Check sheet for the drawn part. Datum: minimum x, y, z corner. Units: mm. A direction names the side the tool comes from. Coordinates: 2 decimals unless noted, no trailing zeros. Order: outer loops, then holes, each group sorted by start corner. A loop starts at its lowest first (then second) coordinate and runs counter-clockwise, first axis right, second up. Notation, with made-up numbers: (0, 19.25) - (4, 19.25) arc R22 cw to (4, 39.25) - close; hole circle Ø7 at (0.5, -8). An arc over 180 degrees is marked (long way). Answer as CSV lines item,"result". Start each with the question number.
1. Section check A-A (x = 6). Record the cut outline in (y, z).
2. Section check C-C (x = 15). Record the cut outline in (y, z).
3. Section check D-D (z = 36). Record the cut outline in (x, y), and give its area (3 significant figures).
4. Section check B-B (y = 17.5). Record the cut outline in (x, z).
5. Set-up check for the marked faces 1 and 2: record each of +Z, -Z, +X, -X, +Y, -Y from which the full face is reachable in a straight line by a thin tool's end or side.
6. Material ranges on L1, parallel to Y at x = 6, z = 46.15; L2, parallel to Z at x = 4, y = 21; L3, parallel to X at y = 29, z = 46, recorded low to high. Write a range as [from, to].
7. Go/stop test with flat-tipped pins: pin 1 (6 mm diameter, centred on x = 19.5, z = 33, fed in from +Y); pin 2 (12 mm diameter, centred on x = 4.5, y = 19.5, fed in from -Z); pin 3 (5 mm diameter, centred on y = 15, z = 38.5, fed in from -X); pin 4 (12 mm diameter, centred on y = 26, z = 42.5, fed in from +X). Record where each tip stops, or that it passes through.
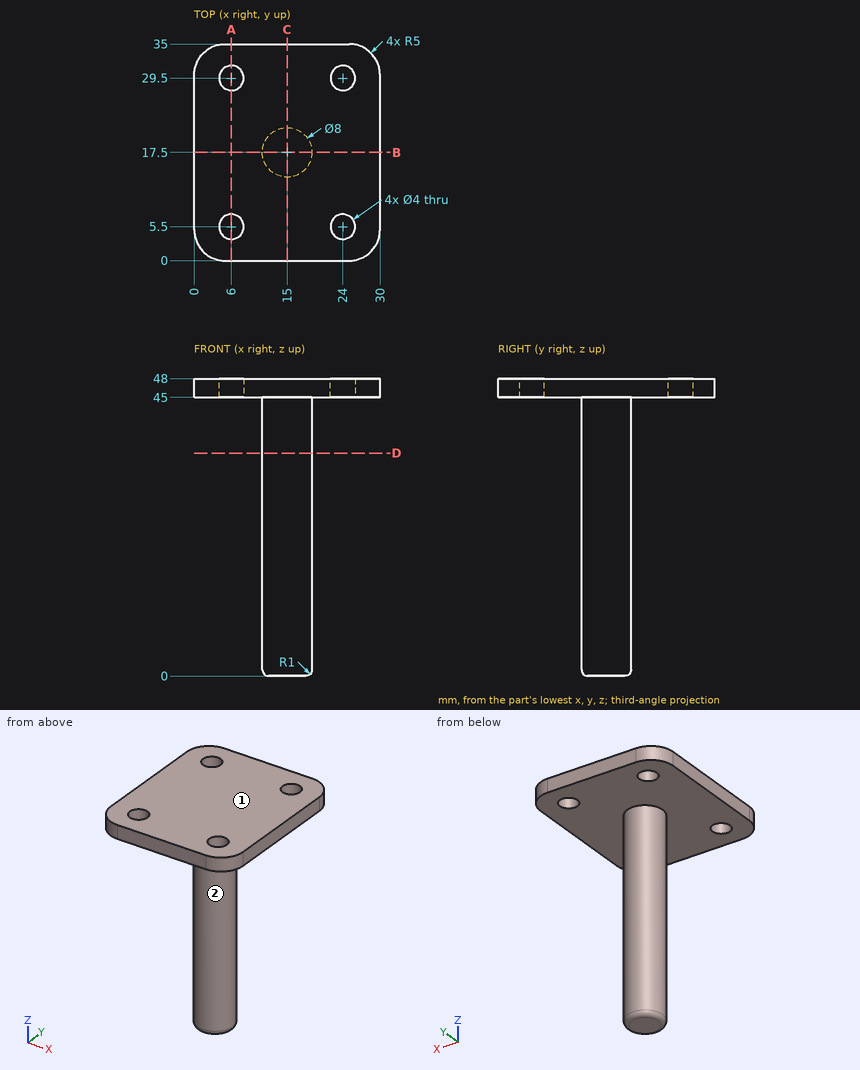
Evaluation:
1,outline,"(0, 45) - (3.5, 45) - (3.5, 48) - (0, 48) - close; (7.5, 45) - (27.5, 45) - (27.5, 48) - (7.5, 48) - close; (31.5, 45) - (35, 45) - (35, 48) - (31.5, 48) - close"
2,outline,"(0, 45) - (13.5, 45) - (13.5, 1) arc R1 ccw to (14.5, 0) - (20.5, 0) arc R1 ccw to (21.5, 1) - (21.5, 45) - (35, 45) - (35, 48) - (0, 48) - close"
3,outline,"circle Ø8 at (15, 17.5)"
3,area,"50.3 mm²"
4,outline,"(0, 45) - (11, 45) - (11, 1) arc R1 ccw to (12, 0) - (18, 0) arc R1 ccw to (19, 1) - (19, 45) - (30, 45) - (30, 48) - (0, 48) - close"
5,face 1,"+Z, +X, -X, +Y, -Y"
5,face 2,"-Z"
6,L1,"y = [0, 3.5], [7.5, 27.5], [31.5, 35]"
6,L2,"z = [45, 48]"
6,L3,"x = [0, 4.06], [7.94, 22.06], [25.94, 30]"
7,pin 1,"stops at y = 21.21"
7,pin 2,"stops at z = 45"
7,pin 3,"stops at x = 11"
7,pin 4,"stops at x = 30"
